Here's how the part is built. I have some questions about the finished solid (model axes, mm). Face numbers are marked on the shaded views. A direction names the side the tool comes from. Give positions to 0.01 mm unless a question says otherwise; leave off trailing zeros. Order: outer loops, then holes, each group sorted by start corner. A loop starts at its lowest first (then second) coordinate and runs counter-clockwise, first axis right, second up. Notation, with made-up numbers: (89.5, 50.5) - (106.5, 50.5) arc R24 ccw to (106.5, 79.5) - close; hole circle Ø8 at (-20.75, -14.5). An arc over 180 degrees is marked (long way). One line per question, with ' | ' between items.
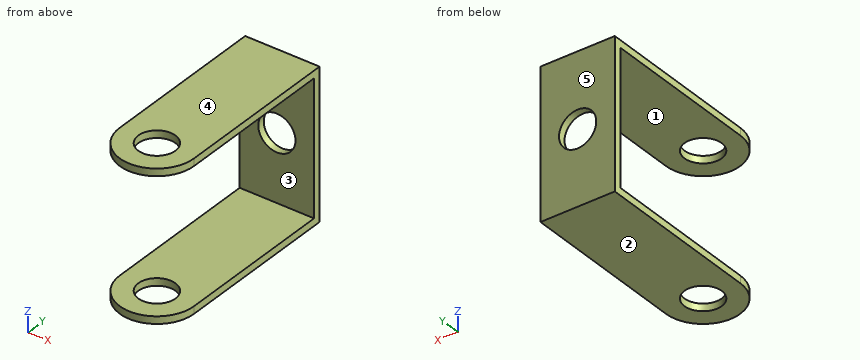
from build123d import *

# Parameters (mm, degrees)
SKETCH1_R           = 12.7
BOSS_EXTRUDE1_DEPTH = 50.8
SKETCH2_W           = 91.6
SKETCH2_H           = 134.7
CUT_EXTRUDE1_DEPTH  = 101.6
SKETCH3_R           = 12.7
CUT_EXTRUDE2_DEPTH  = 101.6


with BuildPart() as part:
    # Sketch1 → Boss-Extrude1 (new, symmetric)
    with BuildSketch(Plane.XY):
        with BuildLine():
            Line((-25.4, 0), (-25.4, 114.3))
            Line((-25.4, 114.3), (25.4, 114.3))
            Line((25.4, 114.3), (25.4, 0))
            ThreePointArc((25.4, 0), (0, -25.4), (-25.4, 0))
        make_face()
        Circle(SKETCH1_R, mode=Mode.SUBTRACT)
    extrude(amount=BOSS_EXTRUDE1_DEPTH, both=True)

    # Sketch2 → Cut-Extrude1 (cut)
    with BuildSketch(Plane(origin=(25.4, 0, 0), x_dir=(0, 0, -1), z_dir=(1, 0, 0))):
        with Locations((0, 41.95)):
            Rectangle(SKETCH2_W, SKETCH2_H)
    extrude(amount=-CUT_EXTRUDE1_DEPTH, mode=Mode.SUBTRACT)

    # Sketch3 → Cut-Extrude2 (cut)
    with BuildSketch(Plane(origin=(0, 114.3, 0), x_dir=(1, 0, 0), z_dir=(0, 1, 0))):
        Circle(SKETCH3_R)
    extrude(amount=-CUT_EXTRUDE2_DEPTH, mode=Mode.SUBTRACT)


solid = part.part
1) I want a section at C-C (z = -10). List the corners of the cut face in (x, y) for me, plus the area to 3 significant figures.
Model answer:
outline: (-25.4, 109.3) - (-7.83, 109.3) - (-7.83, 114.3) - (-25.4, 114.3) - close; (7.83, 109.3) - (25.4, 109.3) - (25.4, 114.3) - (7.83, 114.3) - close | area: 176 mm2
2) Please list where these lines run through material, in increasing order: L1, parallel to X at y = 112, z = 0; L2, parallel to Z at x = 0, y = 112.65; L3, parallel to Y at x = 0, z = -47.15.
Model answer:
L1: x = -25.4 to -12.7, 12.7 to 25.4 | L2: z = -50.8 to -12.7, 12.7 to 50.8 | L3: y = -25.4 to -12.7, 12.7 to 114.3
3) Thinking about a two-plate mould opening in Z: for the marked faces 3, 4 and 5, which applies, +Z half, -Z half, draft (parallel to the pull), parting line (faces both ways), or undercut?
Model answer:
face 3: undercut | face 4: +Z half | face 5: draft
4) I want a section at A-A (y = 82). List the corners of the cut face in (x, z) for me, plus the area to 3 significant figures.
Model answer:
outline: (-25.4, -50.8) - (25.4, -50.8) - (25.4, -45.8) - (-25.4, -45.8) - close; (-25.4, 45.8) - (25.4, 45.8) - (25.4, 50.8) - (-25.4, 50.8) - close | area: 508 mm2
5) I'm going to push flat-ended pins straight in: P1, Ø20.5, axis at x = 0, y = 0, coming from the +Z side; P2, Ø15, axis at x = -7, z = -22, coming from the -Y side. Where does each tip first touch, or does it pass through?
Model answer:
P1: passes through | P2: stops at y = 109.3
6) On a 3-axis mill with a long thin cutter (end or side, diameter ignored), from which of +Z, -Z, +X, -X, +Y, -Y can I reach the whole of each face in a straight line? I mean the marked faces 1 and 2. Say none if no direction works.
Model answer:
face 1: +X, -X, -Y | face 2: -Z, +X, -X, +Y, -Y
7) I want a section at B-B (x = 0). List the corners of the cut face in (y, z) for me.
Model answer:
outline: (-25.4, -50.8) - (-12.7, -50.8) - (-12.7, -45.8) - (-25.4, -45.8) - close; (-25.4, 45.8) - (-12.7, 45.8) - (-12.7, 50.8) - (-25.4, 50.8) - close; (12.7, -50.8) - (114.3, -50.8) - (114.3, -12.7) - (109.3, -12.7) - (109.3, -45.8) - (12.7, -45.8) - close; (12.7, 45.8) - (109.3, 45.8) - (109.3, 12.7) - (114.3, 12.7) - (114.3, 50.8) - (12.7, 50.8) - close
8) I want a section at D-D (y = -9.5). List the corners of the cut face in (x, z) for me, plus the area to 3 significant figures.
Model answer:
outline: (-23.56, -50.8) - (-8.43, -50.8) - (-8.43, -45.8) - (-23.56, -45.8) - close; (-23.56, 45.8) - (-8.43, 45.8) - (-8.43, 50.8) - (-23.56, 50.8) - close; (8.43, -50.8) - (23.56, -50.8) - (23.56, -45.8) - (8.43, -45.8) - close; (8.43, 45.8) - (23.56, 45.8) - (23.56, 50.8) - (8.43, 50.8) - close | area: 303 mm2
